Autodesk Inventor part; units mm, degrees
ref_plane "YZ Plane" through (0, 0, 0) normal (1, 0, 0) x (0, 1, 0)
ref_plane "XZ Plane" through (0, 0, 0) normal (0, 1, 0) x (-1, 0, 0)
ref_plane "XY Plane" through (0, 0, 0) normal (0, 0, 1) x (1, 0, 0)
sketch "Sketch1" plane through (0, 0, 0) normal (0, 1, 0) x (-1, 0, 0)
  circle A0 centre (0, 0) radius 37.5
  circle A1 centre (30, 0) radius 2.75
  circle A2 centre (25.9808, -15) radius 2.75
  circle A3 centre (15, -25.9808) radius 2.75
  circle A4 centre (0, -30) radius 2.75
  circle A5 centre (-15, -25.9808) radius 2.75
  circle A6 centre (-25.9808, -15) radius 2.75
  circle A7 centre (-30, 0) radius 2.75
  circle A8 centre (-25.9808, 15) radius 2.75
  circle A9 centre (-15, 25.9808) radius 2.75
  circle A10 centre (0, 30) radius 2.75
  circle A11 centre (15, 25.9808) radius 2.75
  circle A12 centre (25.9808, 15) radius 2.75
  circle A13 centre (21.0643, 0) radius 5 construction
  dimension "d1" = 5.5
  dimension "d4" = 360
  dimension "d33" = 30
  dimension "d34" = 75
extrude "Extrusion1" add sketch "Sketch1" along normal blind 5
sketch "Sketch2" plane through (0, 5, 0) normal (0, 1, 0) x (1, 0, 0)
  line L0 (0, 0) -> (-49.6447, 0)
  line L1 (0, 0) -> (0, 30.1523)
  line L2 (-17.3205, -10) -> (17.3205, -10)
  line L3 (17.3205, -10) -> (17.3205, -15)
  line L4 (17.3205, -15) -> (-17.3205, -15)
  line L5 (-17.3205, -15) -> (-17.3205, -10)
  line L6 (-17.3205, -10) -> (17.3205, -15) construction
  line L7 (17.3205, -10) -> (-17.3205, -15) construction
  line L8 (-17.3205, 10) -> (17.3205, 10)
  line L9 (17.3205, 10) -> (17.3205, 15)
  line L10 (17.3205, 15) -> (-17.3205, 15)
  line L11 (-17.3205, 15) -> (-17.3205, 10)
  line L12 (-17.3205, 10) -> (17.3205, 15) construction
  line L13 (17.3205, 10) -> (-17.3205, 15) construction
  point P0 (0, -12.5)
  point P1 (0, 12.5)
  dimension "d13" = 20
  dimension "d14" = 34.641
  dimension "d17" = 0
  dimension "d18" = 5
extrude "Extrusion2" add sketch "Sketch2" along normal blind 40
sketch "Sketch4" plane through (-17.3205, 5, 15) normal (0, 0, 1) x (1, 0, 0)
  line L0 (24.8205, 32.5) -> (9.8205, 32.5)
  line L1 (9.8205, 32.5) -> (9.8205, 17.5)
  line L2 (9.8205, 17.5) -> (24.8205, 17.5)
  line L3 (24.8205, 17.5) -> (24.8205, 32.5)
  line L4 (24.8205, 32.5) -> (9.8205, 17.5) construction
  line L5 (9.8205, 32.5) -> (24.8205, 17.5) construction
  line L6 (34.641, 0) -> (34.641, 40)
  line L7 (0, 40) -> (34.641, 40)
  circle A0 centre (9.8205, 32.5) radius 2.75
  circle A1 centre (24.8205, 32.5) radius 2.75
  circle A2 centre (24.8205, 17.5) radius 2.75
  circle A3 centre (9.8205, 17.5) radius 2.75
  point P0 (17.3205, -5)
  point P1 (17.3205, 25)
  dimension "d23" = 15
  dimension "d24" = 17.3205
  dimension "d25" = 15
  dimension "d26" = 15
  dimension "d27" = 5.5
  dimension "d28" = 5.5
  dimension "d29" = 5.5
  dimension "d30" = 5.5
extrude "Extrusion3" cut sketch "Sketch4" against normal blind 80 contours A0 L1 L0 | L0 L1 A0 | A1 L3 L0 | L0 L3 A1 | A3 L2 L1 | L1 L2 A3 | A2 L2 L3 | L3 L2 A2
sketch "Sketch5" plane through (0, 5, 0) normal (0, 1, 0) x (1, 0, 0)
  line L0 (19.8007, 7.1805) -> (-19.8007, 7.1805)
  line L1 (-19.8007, 7.1805) -> (-19.8007, -7.1805)
  line L2 (-19.8007, -7.1805) -> (19.8007, -7.1805)
  line L3 (19.8007, -7.1805) -> (19.8007, 7.1805)
  line L4 (19.8007, 7.1805) -> (-19.8007, -7.1805) construction
  line L5 (-19.8007, 7.1805) -> (19.8007, -7.1805) construction
  point P0 (0, 0)
extrude "Extrusion4" cut sketch "Sketch5" against normal blind 10
properties part number "Base"
Check sheet for the modelled part. Datum: model origin and axes. Units: mm. A direction names the side the tool comes from. Give positions to 0.01 mm unless a question says otherwise; leave off trailing zeros. Write each loop counter-clockwise with the first axis right and the second up, starting at its lowest first coordinate (ties: lowest second). Pieces come first, ordered by that corner, then holes. Notation, with made-up numbers: (22, 2) -> (55, 2) arc R24 ccw to (55, 17) -> close; hole circle Ø3 at (-18, 88). An arc over 180 degrees is marked (long way). One line per item, written item: value. Start each with the question number.
Item 1: Section check A-A on x = 30. Record the cut outline in (y, z).
Item 2: Tool access check on faces 1 (the flat face through (0, 25, 10)), 2 (the flat face through (0, 25, -15)), 3 (the flat face through (19.801, 3, 0)), 4 (the flat face through (17.32, 25, 12)), 5 (the flat face through (-17.32, 25, 13)). Record the directions out of +Z, -Z, +X, -X, +Y, -Y that give a thin tool (end or side, any length) a straight path to the whole face; none if there is none.
Item 3: Section check D-D on z = -14. Record the cut outline in (x, y), then the cut area to 3 significant figures.
Item 4: Section check B-B on z = -30. Record the cut outline in (x, y), then the cut area to 4 significant figures.
Item 5: Draft check along X on faces 6 (the flat face through (1, 5, -8)), 7 (the cylindrical face through (7.142, 40.227, -12.465)), 8 (the cylindrical face through (4.88, 2.46, -37.18)). Enter one of: +X half, -X half, draft (parallel to the pull), parting line (faces both ways), or undercut.
Item 6: Gauge pin test, flat ends, axial feed: pin 1 (6 mm diameter, centred on x = -21, y = 38, fed in from -Z); pin 2 (1.5 mm diameter, centred on y = 25.5, z = -13, fed in from -X); pin 3 (1.5 mm diameter, centred on x = 12.5, y = 28.5, fed in from +Z); pin 4 (1.5 mm diameter, centred on y = 3.5, z = 3, fed in from -X). Record the tip position at first contact, or that the pin passes through.
Item 7: Section check C-C on y = 37.5. Record the cut outline in (x, z).
Item 8: Material ranges on probe 1 along Z at (x, y) = (0, 1); probe 2 along X at (y, z) = (37.5, 13.15); probe 3 along Y at (x, z) = (7.5, 13.9), recorded low to high. Write a range as from..to.
Results list:
1. outline: (0, -22.5) -> (5, -22.5) -> (5, -2.75) -> (0, -2.75) -> close; (0, 2.75) -> (5, 2.75) -> (5, 22.5) -> (0, 22.5) -> close
2. face 1: +X, -X, +Y
2. face 2: -Z, +X, -X, +Y
2. face 3: +Y, -Y
2. face 4: +Z, -Z, +X, +Y
2. face 5: +Z, -Z, -X, +Y
3. outline: (-34.79, 0) -> (-28.54, 0) -> (-28.54, 5) -> (-34.79, 5) -> close; (-23.42, 0) -> (23.42, 0) -> (23.42, 5) -> (17.32, 5) -> (17.32, 45) -> (-17.32, 45) -> (-17.32, 5) -> (-23.42, 5) -> close; (28.54, 0) -> (34.79, 0) -> (34.79, 5) -> (28.54, 5) -> close; hole circle Ø5.5 at (-7.5, 22.5); hole circle Ø5.5 at (-7.5, 37.5); hole circle Ø5.5 at (7.5, 22.5); hole circle Ø5.5 at (7.5, 37.5)
3. area: 1,590 mm²
4. outline: (-22.5, 0) -> (-2.75, 0) -> (-2.75, 5) -> (-22.5, 5) -> close; (2.75, 0) -> (22.5, 0) -> (22.5, 5) -> (2.75, 5) -> close
4. area: 197.5 mm²
5. face 6: draft
5. face 7: undercut
5. face 8: parting line
6. pin 1: through
6. pin 2: x = -17.32
6. pin 3: z = 15
6. pin 4: x = -37.43
7. outline: (-17.32, -15) -> (-10.25, -15) -> (-10.25, -10) -> (-17.32, -10) -> close; (-17.32, 10) -> (-10.25, 10) -> (-10.25, 15) -> (-17.32, 15) -> close; (-4.75, -15) -> (4.75, -15) -> (4.75, -10) -> (-4.75, -10) -> close; (-4.75, 10) -> (4.75, 10) -> (4.75, 15) -> (-4.75, 15) -> close; (10.25, -15) -> (17.32, -15) -> (17.32, -10) -> (10.25, -10) -> close; (10.25, 10) -> (17.32, 10) -> (17.32, 15) -> (10.25, 15) -> close
8. probe 1: -37.5..-32.75, -27.25..-7.18, 7.18..27.25, 32.75..37.5
8. probe 2: -17.32..-10.25, -4.75..4.75, 10.25..17.32
8. probe 3: 0..19.75, 25.25..34.75, 40.25..45
